Geometry check sheet. Reference: drawing and pictorial views, mm from the part's lowest x, y, z. A direction names the side the tool comes from. Round coordinates to 2 decimals unless told otherwise and drop trailing zeros. Order: outer loops, then holes, each group sorted by start corner. A loop starts at its lowest first (then second) coordinate and runs counter-clockwise, first axis right, second up.
(1) Cross-section at A-A on z = 19.05. Enter the section's corners in (x, y).
(2) Gauge pin test, flat ends, axial feed: P1, Ø6, axis at y = 10, z = 40, coming from the +X side; P2, Ø10, axis at y = 20.5, z = 56.5, coming from the -X side; P3, Ø4, axis at x = 8, y = 11, coming from the +Z side. Record the tip position at first contact, or that the pin passes through.
(3) Thickness scan on L1, parallel to Z at x = 44.45, y = 6.75; L2, parallel to X at y = 5, z = 19; L3, parallel to Y at x = 37, z = 10. Record the ranges inside material, lowest first.
(4) Set-up check for the marked faces 5 and 6: record each of +Z, -Z, +X, -X, +Y, -Y from which the full face is reachable in a straight line by a thin tool's end or side.
(5) Draft check along X on the marked faces 1, 2, 3 and 4. Enter one of: pulls with the +X half, pulls with the -X half, needs draft (parallel to the pull), parting line crosses it, or undercut.
(6) Cross-section at D-D on y = 6.5. Enter the section's corners in (x, z), and give its area (3 significant figures).
(7) Cross-section at C-C on x = 44.5. Enter the section's corners in (y, z), and give its area (3 significant figures).
(8) Cross-section at B-B on y = 20. Enter the section's corners in (x, z).
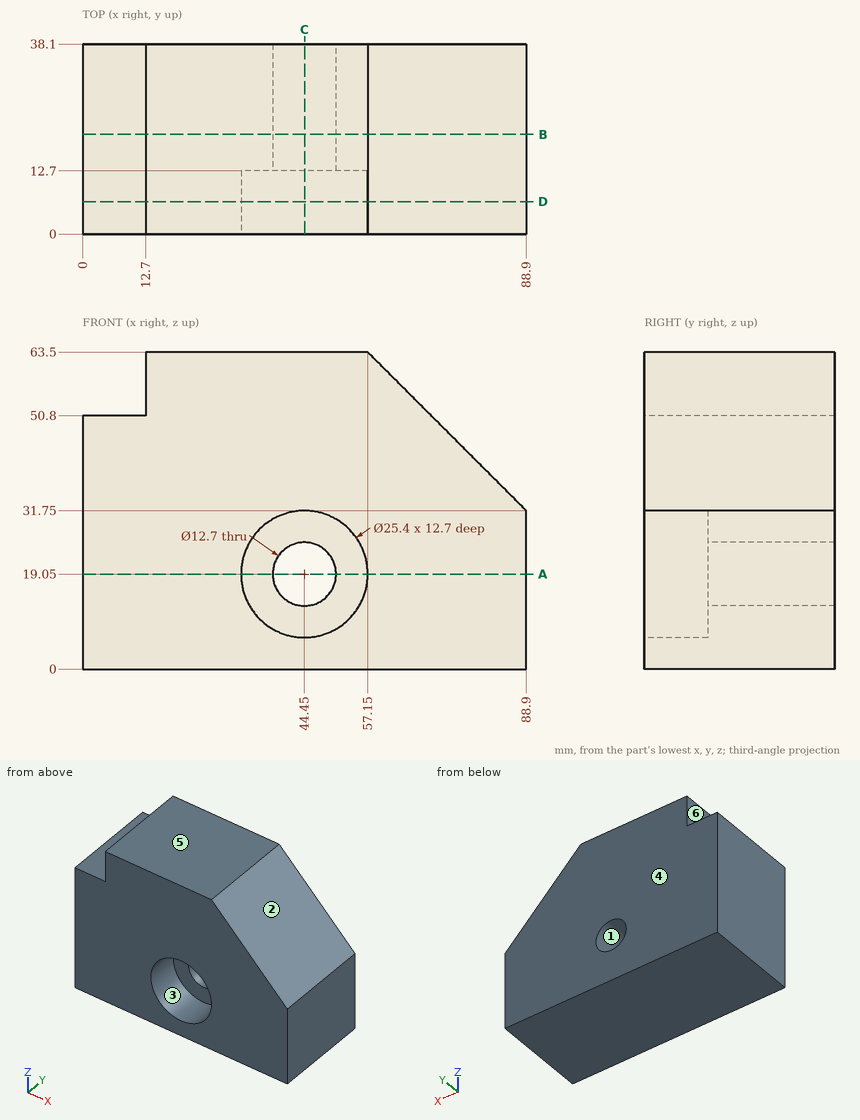
Found:
1. outline: (0, 0) - (31.75, 0) - (31.75, 12.7) - (38.1, 12.7) - (38.1, 38.1) - (0, 38.1) - close; (50.8, 12.7) - (57.15, 12.7) - (57.15, 0) - (88.9, 0) - (88.9, 38.1) - (50.8, 38.1) - close
2. P1: stops at x = 83.65
2. P2: stops at x = 12.7
2. P3: stops at z = 50.8
3. L1: z = 0 to 6.35, 31.75 to 63.5
3. L2: x = 0 to 31.75, 57.15 to 88.9
3. L3: y = 12.7 to 38.1
4. face 5: +Z, +X, -X, +Y, -Y
4. face 6: +Z, -X, +Y, -Y
5. face 1: undercut
5. face 2: pulls with the +X half
5. face 3: undercut
5. face 4: needs draft
6. outline: (0, 0) - (88.9, 0) - (88.9, 31.75) - (57.15, 63.5) - (12.7, 63.5) - (12.7, 50.8) - (0, 50.8) - close; hole circle Ø25.4 at (44.45, 19.05)
6. area: 4,470 mm2
7. outline: (0, 0) - (38.1, 0) - (38.1, 12.7) - (12.7, 12.7) - (12.7, 6.35) - (0, 6.35) - close; (0, 31.75) - (12.7, 31.75) - (12.7, 25.4) - (38.1, 25.4) - (38.1, 63.5) - (0, 63.5) - close
7. area: 1,770 mm2
8. outline: (0, 0) - (88.9, 0) - (88.9, 31.75) - (57.15, 63.5) - (12.7, 63.5) - (12.7, 50.8) - (0, 50.8) - close; hole circle Ø12.7 at (44.45, 19.05)
